```python
from build123d import *

# Parameters (mm, degrees)
SKETCH1_R           = 30
BOSS_EXTRUDE1_DEPTH = 25
SKETCH2_R           = 12.5
CUT_EXTRUDE1_DEPTH  = 10
FILLET1_R           = 5
FILLET2_R           = 7


with BuildPart() as part:
    # Sketch1 → Boss-Extrude1 (new body)
    with BuildSketch(Plane.XY):
        Circle(SKETCH1_R)
    extrude(amount=BOSS_EXTRUDE1_DEPTH)

    # Sketch2 → Cut-Extrude1 (cut)
    with BuildSketch(Plane.XY.offset(25)):
        Circle(SKETCH2_R)
    extrude(amount=-CUT_EXTRUDE1_DEPTH, mode=Mode.SUBTRACT)

    # Fillet1
    fillet1_edges = [part.edges().sort_by_distance(p)[0] for p in [
        (-12.5, 0, 15),
        (-12.5, 0, 25),
    ]]
    fillet(fillet1_edges, radius=FILLET1_R - 0.0001)  # a hair under: the kernel refuses the full size

    # Fillet2
    fillet2_edges = [part.edges().sort_by_distance(p)[0] for p in [
        (-30, 0, 0),
        (-30, 0, 25),
    ]]
    fillet(fillet2_edges, radius=FILLET2_R)


solid = part.part
```
Verification items for the finished model (mm, model axes). Coordinates: 2 decimals unless noted, no trailing zeros. Loops run counter-clockwise (first coordinate to the right, second up) from the corner with the lowest first, then second, coordinate; pieces in that order, holes last. Notation, with made-up numbers: (-3.75, -39) - (44.25, -39) arc R26 ccw to (44.25, -15) - close; hole circle Ø7 at (14.25, 36). An arc over 180 degrees is marked (long way). Answer as a JSON object with one key per item and string values.
(1) Scan lines: line 1 along Y through (x, z) = (0, 20); line 2 along Z through (x, y) = (16, 17); line 3 along Y through (x, z) = (17, 13.25). Record each from-to range of solid material in increasing order.
Response:
{"line 1": "y = -29.71 to -12.5, 12.5 to 29.71", "line 2": "z = 0.01 to 24.99", "line 3": "y = -24.72 to 24.72"}
(2) Cross-section at C-C, the plane z = 23.25. Record the boundary of the cut face in (x, y).
Response:
{"outline": "circle Ø55.26 at (0, 0); hole circle Ø27.4 at (0, 0)"}
(3) Cross-section at D-D, the plane z = 8.5. Record the boundary of the cut face in (x, y).
Response:
{"outline": "circle Ø60 at (0, 0)"}
(4) Go/stop test with flat-tipped pins: pin 1 Ø1 at (x, z) = (-10, 13.5) entering from -Y; pin 2 Ø10 at (x, z) = (-6, 13.5) entering from +Y; pin 3 Ø4.5 at (x, y) = (3.5, 2.5) entering from +Z. Record where each tip stops, or that it passes through.
Response:
{"pin 1": "stops at y = -28.46", "pin 2": "stops at y = 29.98", "pin 3": "stops at z = 15"}
(5) Mould release check, pull along X, two halves, no side actions. Record for faces 1 (the flat face through (0, 0, 0)), 2 (the cylindrical face through (-29.97, 1.32, 12.42)), 3 (the flat face through (0, 0, 15)): pulls with the +X half, pulls with the -X half, needs draft (parallel to the pull), parting line crosses it, or undercut.
Response:
{"face 1": "needs draft", "face 2": "parting line crosses it", "face 3": "undercut"}
